from build123d import *

# Parameters (mm, degrees)
FILLET_1_R               = 1
EXTRUDE_START            = -19.4
EXTRUDE_1_DEPTH          = 19.4
CUT_EXTRUDE_8_DEPTH      = 45.932997117
CUT_EXTRUDE_8_DEPTH_BACK = 45.932997117


with BuildPart() as part:
    # 草图1 → 旋转1 (revolve)
    with BuildSketch(Plane.XY, mode=Mode.PRIVATE) as revolve_1_sk:
        Polygon((2, 15), (2, 0), (2.75, 0), (2.75, 10), (4.65, 10), (4.65, 31.4), (3.2, 31.4), (3.2, 44.4), (2.2, 44.4), (2.2, 26.4), (2.65, 26.4), (2.65, 15), align=None)
    revolve(revolve_1_sk.sketch.rotate(Axis((0, -4.665178571, 0), (0, 1, 0)), 90), axis=Axis((0, -4.665178571, 0), (0, 1, 0)))

    # 圆角1
    # the kernel refuses this fillet: 1 mm, written as the material it takes off along each edge
    with BuildSketch(Plane(origin=(0, 31.4, 0), x_dir=(0, 0, -1), z_dir=(1, 0, 0))) as fillet_1_piece_1:
        with BuildLine():
            CenterArc((4.65 - FILLET_1_R, -FILLET_1_R), FILLET_1_R, 0, 90)
            Line((4.65 - FILLET_1_R, 0), (4.65 - FILLET_1_R, FILLET_1_R * 0.02))
            Line((4.65 - FILLET_1_R, FILLET_1_R * 0.02), (4.65 + FILLET_1_R * 0.02, FILLET_1_R * 0.02))
            Line((4.65 + FILLET_1_R * 0.02, FILLET_1_R * 0.02), (4.65 + FILLET_1_R * 0.02, -FILLET_1_R))
            Line((4.65 + FILLET_1_R * 0.02, -FILLET_1_R), (4.65, -FILLET_1_R))
        make_face()
    revolve(axis=Axis((0, 31.4, 0), (0, 1, 0)), mode=Mode.SUBTRACT)
    with BuildSketch(Plane(origin=(0, 10, 0), x_dir=(0, 0, -1), z_dir=(1, 0, 0))) as fillet_1_piece_2:
        with BuildLine():
            CenterArc((4.65 - FILLET_1_R, FILLET_1_R), FILLET_1_R, 270, 90)
            Line((4.65, FILLET_1_R), (4.65 + FILLET_1_R * 0.02, FILLET_1_R))
            Line((4.65 + FILLET_1_R * 0.02, FILLET_1_R), (4.65 + FILLET_1_R * 0.02, -FILLET_1_R * 0.02))
            Line((4.65 + FILLET_1_R * 0.02, -FILLET_1_R * 0.02), (4.65 - FILLET_1_R, -FILLET_1_R * 0.02))
            Line((4.65 - FILLET_1_R, -FILLET_1_R * 0.02), (4.65 - FILLET_1_R, 0))
        make_face()
    revolve(axis=Axis((0, 10, 0), (0, 1, 0)), mode=Mode.SUBTRACT)
    with BuildSketch(Plane(origin=(0, 0, 0), x_dir=(0, 0, -1), z_dir=(1, 0, 0))) as fillet_1_piece_3:
        with BuildLine():
            CenterArc((1.75, 0.968245837), FILLET_1_R, 284.477512186, 75.522487814)
            Line((2.75, 0.968245837), (2.77, 0.968245837))
            Line((2.77, 0.968245837), (2.77, 0))
            Line((2.77, 0), (2.75, -0.02))
            ThreePointArc((2.75, -0.02), (2.375, -0.02), (2.005, -0.019364917))
            Line((2.005, -0.019364917), (2, 0))
        make_face()
    revolve(axis=Axis((0, 0, 0), (0, 1, 0)), mode=Mode.SUBTRACT)

    # 草图2 → 凸台-拉伸1 (add)
    with BuildSketch(Plane(origin=(0, 30.4, 0), x_dir=(1, 0, 0), z_dir=(0, 1, 0)).offset(EXTRUDE_START)):
        with BuildLine():
            Line((2.779213221, 3.728065701), (1.234997781, 4.879253527))
            Line((1.234997781, 4.879253527), (-0.670940138, 4.601341036))
            ThreePointArc((-0.670940138, 4.601341036), (1.140989177, 4.507842466), (2.779213221, 3.728065701))
        make_face()
        with BuildLine():
            ThreePointArc((-3.728065726, 2.779213188), (-2.38072481, 3.99432715), (-0.670940138, 4.601341036))
            Line((-0.670940138, 4.601341036), (-2.57687795, 4.323428561))
            Line((-2.57687795, 4.323428561), (-3.728065726, 2.779213188))
        make_face()
        with BuildLine():
            Line((4.323428561, 2.57687795), (2.779213221, 3.728065701))
            ThreePointArc((2.779213221, 3.728065701), (3.994327171, 2.380724774), (4.601341042, 0.670940096))
            Line((4.601341042, 0.670940096), (4.323428561, 2.57687795))
        make_face()
        with BuildLine():
            ThreePointArc((-4.601341043, -0.67094009), (-4.507842465, 1.14098918), (-3.728065726, 2.779213188))
            Line((-3.728065726, 2.779213188), (-4.879253527, 1.234997781))
            Line((-4.879253527, 1.234997781), (-4.601341043, -0.67094009))
        make_face()
        with BuildLine():
            Line((4.879253527, -1.234997781), (4.601341042, 0.670940096))
            ThreePointArc((4.601341042, 0.670940096), (4.50784246, -1.1409892), (3.728065698, -2.779213226))
            Line((3.728065698, -2.779213226), (4.879253527, -1.234997781))
        make_face()
        with BuildLine():
            ThreePointArc((-2.779213228, -3.728065696), (-3.994327175, -2.380724768), (-4.601341043, -0.67094009))
            Line((-4.601341043, -0.67094009), (-4.323428561, -2.57687795))
            Line((-4.323428561, -2.57687795), (-2.779213228, -3.728065696))
        make_face()
        with BuildLine():
            ThreePointArc((0.670940034, -4.601341051), (-1.140989232, -4.507842452), (-2.779213228, -3.728065696))
            Line((-2.779213228, -3.728065696), (-1.234997781, -4.879253527))
            Line((-1.234997781, -4.879253527), (0.670940034, -4.601341051))
        make_face()
        with BuildLine():
            Line((2.57687795, -4.323428561), (3.728065698, -2.779213226))
            ThreePointArc((3.728065698, -2.779213226), (2.380724745, -3.994327189), (0.670940034, -4.601341051))
            Line((0.670940034, -4.601341051), (2.57687795, -4.323428561))
        make_face()
    extrude(amount=EXTRUDE_1_DEPTH)

    # 草图3 → 切除-拉伸8 (cut, two sides: drawn at the far end of the back side and taken through both)
    with BuildSketch(Plane.XY.offset(-CUT_EXTRUDE_8_DEPTH_BACK)):
        Polygon((-3.65, 42.874542092), (-3.65, 41.874542092), (-3.2, 41.874542092), (-1.7, 41.874542092), (-1.7, 42.874542092), (-3.2, 42.874542092), (-3.263750078, 42.874542092), align=None)
        Polygon((-3.65, 39.16171454), (-3.65, 38.513443063), (-3.2, 38.513443063), (-1.960187726, 38.513443063), (-1.960187726, 39.16171454), (-3.2, 39.16171454), align=None)
        Polygon((-3.65, 34.063943377), (-3.2, 34.063943377), (-1.960187726, 34.063943377), (-1.960187726, 35.006883708), (-3.2, 35.006883708), (-3.65, 35.006883708), align=None)
        Polygon((3.2, 36.097158465), (3.65, 36.097158465), (3.65, 37.040098796), (3.2, 37.040098796), (2.017841794, 37.040098796), (2.017841794, 36.097158465), align=None)
        Polygon((3.2, 39.751052247), (3.65, 39.751052247), (3.65, 41.077062087), (3.2, 41.077062087), (2.017841794, 41.077062087), (2.017841794, 39.751052247), align=None)
        Polygon((3.2, 32.384330913), (3.65, 32.384330913), (3.65, 33.209403702), (3.277688682, 33.209403702), (3.2, 33.209403702), (2.017841794, 33.209403702), (2.017841794, 32.384330913), align=None)
    extrude(amount=CUT_EXTRUDE_8_DEPTH + CUT_EXTRUDE_8_DEPTH_BACK, mode=Mode.SUBTRACT)


solid = part.part
Check sheet for the modelled part. Datum: model origin and axes. Units: mm. A direction names the side the tool comes from. Round coordinates to 2 decimals unless told otherwise and drop trailing zeros. Loops run counter-clockwise (first coordinate to the right, second up) from the corner with the lowest first, then second, coordinate; pieces in that order, holes last. Notation, with made-up numbers: (-37.75, 35.25) -> (4.25, 35.25) arc R12 cw to (4.25, 46.25) -> close; hole circle Ø11 at (-16.75, 0.25). An arc over 180 degrees is marked (long way). Put each result on its own line as item: value. Start each with the question number.
1. Scan lines: probe 1 along X at (y, z) = (7.75, 0); probe 2 along Y at (x, z) = (-1, -3.25); probe 3 along Z at (x, y) = (-1.25, 29.5). Record each from-to range of solid material in increasing order.
2. Section check A-A (y = 16). Enter the section's corners in (x, z) (3 decimals), plus the area to 3 significant figures.
3. Draft check along Y on faces 4 (the face through (4.7, 30.4, 1.2)), 5 (the face through (2.018, 40, -2)), 6 (the face through (1.2, 11, -4.7)). Enter one of: +Y half, -Y half, draft (parallel to the pull), parting line (faces both ways), or undercut.
4. Access from +Z, -Z, +X, -X, +Y, -Y to the whole of each face (thin tool, end or side, straight path). Record for faces 1 (the face through (2.018, 36.6, -1.7)), 2 (the face through (-1.7, 42.4, -2.1)), 3 (the face through (-2.43, 30.4, -4.17)).
5. Section check C-C (y = 30). Enter the section's corners in (x, z) (3 decimals).
6. Section check D-D (z = 0). Give the number of separate pieces and of enclosed holes in the cut face, plus the area to 3 significant figures.
7. Gauge pin test, flat ends, axial feed: pin 1 (0.5 mm diameter, centred on y = 39, z = 1.5, fed in from -X); pin 2 (0.9 mm diameter, centred on x = 0.5, z = -4.5, fed in from -Y); pin 3 (0.5 mm diameter, centred on y = 34.5, z = 1.5, fed in from -X); pin 4 (5 mm diameter, centred on y = 14.5, z = 3.5, fed in from +X). Record the tip position at first contact, or that the pin passes through.
Findings:
1. probe 1: x = -2.75 to -2, 2 to 2.75
1. probe 2: y = 10 to 31.4
1. probe 3: z = -4.52 to -1.81, 1.81 to 4.87
2. outline: (-4.879, -1.235) -> (-2.577, -4.323) -> (1.235, -4.879) -> (4.323, -2.577) -> (4.879, 1.235) -> (2.577, 4.323) -> (-1.235, 4.879) -> (-4.323, 2.577) -> close; hole circle Ø5.3 at (0, 0)
2. area: 49.6 mm^2
3. face 4: +Y half
3. face 5: undercut
3. face 6: -Y half
4. face 1: +Z, -Z, +X
4. face 2: +Z, -Z, -X
4. face 3: -Z, -X, +Y
5. outline: (-4.879, -1.235) -> (-2.577, -4.323) -> (1.235, -4.879) -> (4.323, -2.577) -> (4.879, 1.235) -> (2.577, 4.323) -> (-1.235, 4.879) -> (-4.323, 2.577) -> close; hole circle Ø4.4 at (0, 0)
6. separate pieces: 8
6. enclosed holes: 0
6. area: 133 mm^2
7. pin 1: stops at x = -2.92
7. pin 2: stops at y = 10.1
7. pin 3: stops at x = -1.96
7. pin 4: stops at x = 4.88
